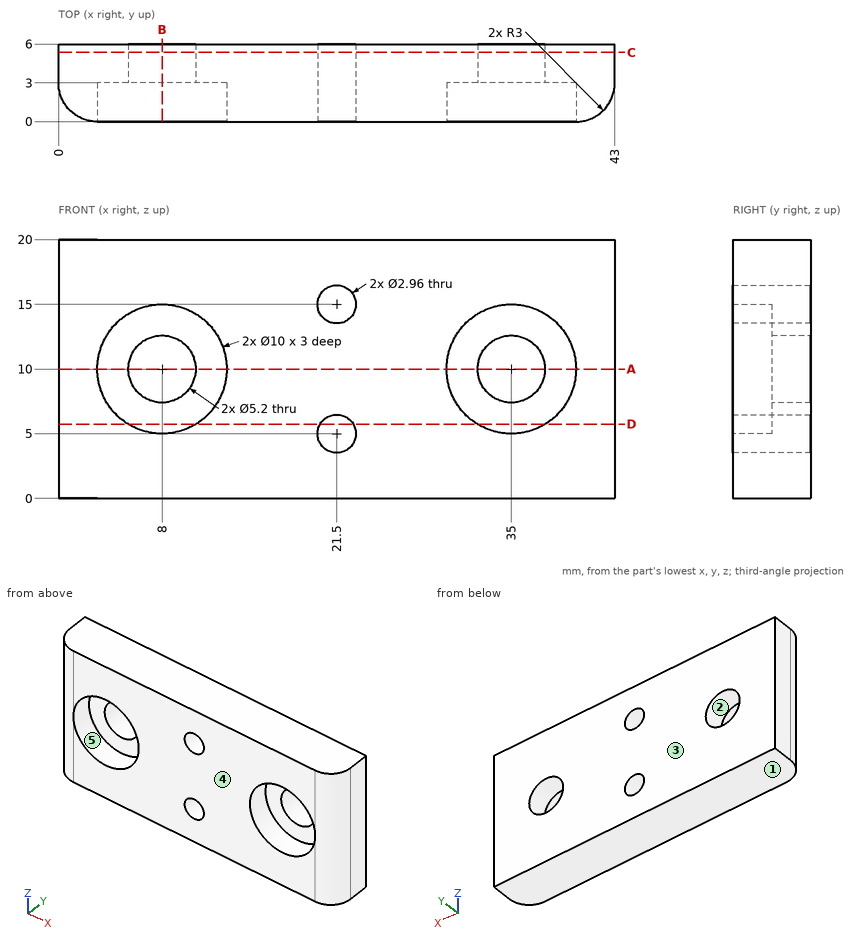
Geometry: see drawing. Coordinates: mm, zero at the bounding-box minimum. A direction names the side the tool comes from. Round coordinates to 2 decimals unless told otherwise and drop trailing zeros. Loops run counter-clockwise (first coordinate to the right, second up) from the corner with the lowest first, then second, coordinate; pieces in that order, holes last. Notation, with made-up numbers: M 87.25,-37 L 143.25,-37 A26 ccw 143.25,-1 Z; hole C 44,88.5 d3. An arc over 180 degrees is marked long. Use a Markdown table: item, result. Add a question column.
1. Mould query, pull axis Z, two halves, no side actions, for the marked faces 1, 2 and 3. Classes: pulls with the +Z half, pulls with the -Z half, needs draft (parallel to the pull), parting line crosses it, or undercut.
2. Reachability of the marked faces 4 and 5 from +Z, -Z, +X, -X, +Y, -Y: full face, straight path, thin tool, end or side. Return the list, or none.
3. Section query A-A on z = 10. Give the number of separate pieces and of enclosed holes in the cut face, then the cut area to 3 significant figures.
4. Section query B-B on x = 8. Return the cut outline in (y, z).
5. Section query D-D on z = 5.75. Return the cut outline in (x, y).
6. Contact query for a flat-ended pin moving along its axis: P1, Ø5, axis at x = 33, z = 12, coming from the -Y side. Output: stop coordinate, or through.
7. Line query: line 1 (X direction, y = 3.4, z = 8.75); line 2 (X direction, y = 3.15, z = 5); line 3 (X direction, y = 1.3, z = 8.25). Output: solid intervals per line, ascending.
8. Section query C-C on y = 5.35. Return the cut outline in (x, z), then the cut area to 3 significant figures.
Reported:
| question | item | result |
|---|---|---|
| 1 | face 1 | pulls with the -Z half |
| 1 | face 2 | undercut |
| 1 | face 3 | needs draft |
| 2 | face 4 | +Z, -Z, +X, -X, -Y |
| 2 | face 5 | -Y |
| 3 | separate pieces | 3 |
| 3 | enclosed holes | 0 |
| 3 | area | 163 mm² |
| 4 | outline | M 0,0 L 6,0 L 6,7.4 L 3,7.4 L 3,5 L 0,5 Z; M 0,15 L 3,15 L 3,12.6 L 6,12.6 L 6,20 L 0,20 Z |
| 5 | outline | M 0,3 A3 ccw 3,0 L 5.37,0 L 5.37,3 L 10.63,3 L 10.63,0 L 20.22,0 L 20.22,6 L 0,6 Z; M 22.78,0 L 32.37,0 L 32.37,3 L 37.63,3 L 37.63,0 L 40,0 A3 ccw 43,3 L 43,6 L 22.78,6 Z |
| 6 | P1 | stops at y = 0 |
| 7 | line 1 | x = 0 to 5.72, 10.28 to 32.72, 37.28 to 43 |
| 7 | line 2 | x = 0 to 20.02, 22.98 to 43 |
| 7 | line 3 | x = 0.53 to 3.32, 12.68 to 30.32, 39.68 to 42.47 |
| 8 | outline | M 0,0 L 43,0 L 43,20 L 0,20 Z; hole C 8,10 d5.2; hole C 21.5,5 d2.96; hole C 21.5,15 d2.96; hole C 35,10 d5.2 |
| 8 | area | 804 mm² |
